Source: CAD feature listing. Evaluate the final solid. Frame: model axes, mm. A direction names the side the tool comes from. Give positions to 0.01 mm unless a question says otherwise; leave off trailing zeros. Write each loop counter-clockwise with the first axis right and the second up, starting at its lowest first coordinate (ties: lowest second). Pieces come first, ordered by that corner, then holes. Notation, with made-up numbers: (54, -37) -> (107, -37) arc R20 ccw to (107, -25) -> close; hole circle Ø3 at (34, 87). An arc over 180 degrees is marked (long way). Answer as a JSON object with one key per item and string values. Group by question number.
Item 1: Section query B-B on x = -9.45. Return the cut outline in (y, z).
Item 2: Ray query, probe 1 along Y at (x, z) = (11.55, -0.75); probe 2 along Y at (x, z) = (0.75, -0.7); probe 3 along Y at (x, z) = (-2.5, 0.6). Return the intervals inside material, ascending. Write a range as from..to.
Item 3: Section query C-C on x = -4.75. Return the cut outline in (y, z), plus the area to 3 significant figures.
Item 4: Access query for faces 1 (the face through (-2, -1, 0)), 2 (the face through (-0.292, 22, -1)), 3 (the face through (-13, 0, -1.2)). Directions: +Z, -Z, +X, -X, +Y, -Y. A direction counts if a zero-diameter tool reaches every point of the face in a straight line with its end or side. Return the directions, or none.
Item 5: Pull-direction query (Y, two-part tool) for faces 4 (the face through (0, 32.8, -1)), 5 (the face through (2, -31.334, -1)), 6 (the face through (10, 27, -2.2)); classes: pulls with the +Y half, pulls with the -Y half, needs draft (parallel to the pull), parting line crosses it, or undercut.
Item 6: First-contact query: pin 1 Ø0.6 at (x, z) = (0.5, -0.5) entering from -Y; pin 2 Ø10 at (x, y) = (1.5, -23) entering from +Z; pin 3 Ø4 at (x, y) = (-2, -22) entering from -Z; pin 4 Ø1.9 at (x, y) = (0.5, 0) entering from +Z. Flat tips, straight axial feed; report the tip coordinate or a pass-through.
from build123d import *

# Parameters (mm, degrees)
SKETCH_2_W          = 29.1
SKETCH_2_H          = 67.8
EXTRUDE_1_DEPTH     = 0.8
SKETCH_3_W          = 29.1
SKETCH_3_H          = 65.6
EXTRUDE_2_DEPTH     = 1.2
SKETCH_4_R          = 1.4
SKETCH_4_W          = 7.042
SKETCH_4_H          = 18.5736
SKETCH_4_W_2        = 4.2
SKETCH_4_H_2        = 8.9
SKETCH_4_W_3        = 8.32
SKETCH_4_H_3        = 15.7
CUT_EXTRUDE_1_DEPTH = 37.944722221
SKETCH_5_R          = 2.1
SKETCH_5_R_2        = 1.1
SKETCH_5_R_3        = 1
EXTRUDE_3_DEPTH     = 1
SKETCH_6_W          = 1
SKETCH_6_H          = 65.6
EXTRUDE_4_DEPTH     = 1
CHAMFER_1_SIZE      = 1
CHAMFER_3_SIZE      = 1
SKETCH_7_W          = 9.042
SKETCH_7_H          = 20.5736
SKETCH_7_W_2        = 6.2
SKETCH_7_H_2        = 10.9
SKETCH_7_W_3        = 10.32
SKETCH_7_H_3        = 17.7
CUT_EXTRUDE_2_DEPTH = 0.8
FILLET_3_R          = 0.8
FILLET_4_R          = 0.8
FILLET_5_R          = 0.8
SKETCH_8_R          = 1.4
CUT_EXTRUDE_3_DEPTH = 37.944722221
CHAMFER_4_SIZE      = 0.6
FILLET_6_R          = 1.6


with BuildPart() as part:
    # Эскиз2 → Бобышка-Вытянуть1 (new body)
    with BuildSketch(Plane.XY):
        Rectangle(SKETCH_2_W, SKETCH_2_H)
    extrude(amount=EXTRUDE_1_DEPTH)

    # Эскиз3 → Бобышка-Вытянуть2 (add)
    with BuildSketch(Plane(origin=(0, 0, 0), x_dir=(-1, 0, 0), z_dir=(0, 0, -1))):
        Rectangle(SKETCH_3_W, SKETCH_3_H)
    extrude(amount=EXTRUDE_2_DEPTH)

    # Эскиз4 → Вырез-Вытянуть1 (cut, through all)
    with BuildSketch(Plane.XY.offset(0.8)):
        with Locations((-9.45, -27.9)):
            Circle(SKETCH_4_R)
        with Locations((11.55, -27.9)):
            Circle(SKETCH_4_R)
        with Locations((11.55, 27.9)):
            Circle(SKETCH_4_R)
        with Locations((-9.45, 27.9)):
            Circle(SKETCH_4_R)
        with Locations((3.229, 22.395)):
            Rectangle(SKETCH_4_W, SKETCH_4_H)
        with Locations((0.55, -0.961534596)):
            Rectangle(SKETCH_4_W_2, SKETCH_4_H_2)
        with Locations((1.86, -23.483733333)):
            Rectangle(SKETCH_4_W_3, SKETCH_4_H_3)
    extrude(amount=-CUT_EXTRUDE_1_DEPTH, mode=Mode.SUBTRACT)

    # Эскиз5 → Бобышка-Вытянуть3 (add)
    # profile 1 of 4: a face of its own
    with BuildSketch(Plane(origin=(0, 0, -1.2), x_dir=(-1, 0, 0), z_dir=(0, 0, -1))):
        with Locations((-11.55, 27.9)):
            Circle(SKETCH_5_R)
        with Locations((-11.55, 27.9)):
            Circle(SKETCH_5_R_2, mode=Mode.SUBTRACT)
    # profile 2 of 4: a face of its own
    with BuildSketch(Plane(origin=(0, 0, -1.2), x_dir=(-1, 0, 0), z_dir=(0, 0, -1))):
        with Locations((-11.55, -27.9)):
            Circle(SKETCH_5_R)
        with Locations((-11.55, -27.9)):
            Circle(SKETCH_5_R_2, mode=Mode.SUBTRACT)
    # profile 3 of 4: a face of its own
    with BuildSketch(Plane(origin=(0, 0, -1.2), x_dir=(-1, 0, 0), z_dir=(0, 0, -1))):
        with Locations((9.45, 27.9)):
            Circle(SKETCH_5_R)
        with Locations((9.45, 27.9)):
            Circle(SKETCH_5_R_3, mode=Mode.SUBTRACT)
    # profile 4 of 4: a face of its own
    with BuildSketch(Plane(origin=(0, 0, -1.2), x_dir=(-1, 0, 0), z_dir=(0, 0, -1))):
        with Locations((9.45, -27.9)):
            Circle(SKETCH_5_R)
        with Locations((9.45, -27.9)):
            Circle(SKETCH_5_R_3, mode=Mode.SUBTRACT)
    extrude(amount=EXTRUDE_3_DEPTH)

    # Эскиз6 → Бобышка-Вытянуть4 (add)
    with BuildSketch(Plane(origin=(0, 0, -1.2), x_dir=(-1, 0, 0), z_dir=(0, 0, -1))):
        with Locations((11.95, 0)):
            Rectangle(SKETCH_6_W, SKETCH_6_H)
    extrude(amount=EXTRUDE_4_DEPTH)

    # Фаска1
    chamfer_1_edges = [part.edges().sort_by_distance(p)[0] for p in [
        (-11.95, -32.8, -2.2),
        (-11.95, 32.8, -2.2),
    ]]
    chamfer(chamfer_1_edges, length=CHAMFER_1_SIZE)

    # Фаска3
    chamfer_3_edges = [part.edges().sort_by_distance(p)[0] for p in [
        (-11.45, -30.670156212, -1.2),
        (-11.45, 30.670156212, -1.2),
        (-11.45, 0, -1.2),
    ]]
    chamfer(chamfer_3_edges, length=CHAMFER_3_SIZE - 0.0001)  # a hair under: the kernel refuses the full size

    # Эскиз7 → Вырез-Вытянуть2 (cut)
    with BuildSketch(Plane.XY.offset(0.8)):
        with Locations((3.229, 22.395)):
            Rectangle(SKETCH_7_W, SKETCH_7_H)
        with Locations((0.55, -0.961534596)):
            Rectangle(SKETCH_7_W_2, SKETCH_7_H_2)
        with Locations((1.86, -23.483733333)):
            Rectangle(SKETCH_7_W_3, SKETCH_7_H_3)
    extrude(amount=-CUT_EXTRUDE_2_DEPTH, mode=Mode.SUBTRACT)

    # Скругление3
    fillet_3_edges = [part.edges().sort_by_distance(p)[0] for p in [
        (3.229, 12.1082, 0.8),
        (7.75, 22.395, 0.8),
        (3.229, 32.6818, 0.8),
        (-1.292, 22.395, 0.8),
    ]]
    fillet(fillet_3_edges, radius=FILLET_3_R - 0.0001)  # a hair under: the kernel refuses the full size

    # Скругление4
    fillet_4_edges = [part.edges().sort_by_distance(p)[0] for p in [
        (0.55, -6.411534596, 0.8),
        (-2.55, -0.961534596, 0.8),
        (0.55, 4.488465404, 0.8),
        (3.65, -0.961534596, 0.8),
    ]]
    fillet(fillet_4_edges, radius=FILLET_4_R - 0.0001)  # a hair under: the kernel refuses the full size

    # Скругление5
    fillet_5_edges = [part.edges().sort_by_distance(p)[0] for p in [
        (1.86, -32.333733333, 0.8),
        (-3.3, -23.483733333, 0.8),
        (1.86, -14.633733333, 0.8),
        (7.02, -23.483733333, 0.8),
    ]]
    fillet(fillet_5_edges, radius=FILLET_5_R - 0.0001)  # a hair under: the kernel refuses the full size

    # Эскиз8 → Вырез-Вытянуть3 (cut, through all)
    with BuildSketch(Plane.XY.offset(-1.2)):
        with Locations((11.55, 27.9)):
            Circle(SKETCH_8_R)
        with Locations((-9.45, -27.9)):
            Circle(SKETCH_8_R)
        with Locations((11.55, -27.9)):
            Circle(SKETCH_8_R)
        with Locations((-9.45, 27.9)):
            Circle(SKETCH_8_R)
    extrude(amount=-CUT_EXTRUDE_3_DEPTH, mode=Mode.SUBTRACT)

    # Фаска4
    chamfer_4_edges = [part.edges().sort_by_distance(p)[0] for p in [
        (10.15, -27.9, 0.8),
        (10.15, 27.9, 0.8),
        (-10.85, 27.9, 0.8),
        (-10.85, -27.9, 0.8),
    ]]
    chamfer(chamfer_4_edges, length=CHAMFER_4_SIZE)

    # Скругление6
    fillet_6_edges = [part.edges().sort_by_distance(p)[0] for p in [
        (-14.55, 0, 0.8),
    ]]
    fillet(fillet_6_edges, radius=FILLET_6_R)


solid = part.part
Worked answers:
{
 "1": {"outline": "(-33.9, 0) -> (-32.8, 0) -> (-32.8, -1.2) -> (-30, -1.2) -> (-30, -2.2) -> (-29.3, -2.2) -> (-29.3, 0.2) -> (-29.9, 0.8) -> (-33.9, 0.8) -> close; (-26.5, -2.2) -> (-25.8, -2.2) -> (-25.8, -1.2) -> (25.8, -1.2) -> (25.8, -2.2) -> (26.5, -2.2) -> (26.5, 0.2) -> (25.9, 0.8) -> (-25.9, 0.8) -> (-26.5, 0.2) -> close; (29.3, -2.2) -> (30, -2.2) -> (30, -1.2) -> (32.8, -1.2) -> (32.8, 0) -> (33.9, 0) -> (33.9, 0.8) -> (29.9, 0.8) -> (29.3, 0.2) -> close"},
 "2": {"probe 1": "-32.8..-29.3, -26.5..26.5, 29.3..32.8", "probe 2": "-32.8..-31.33, -15.63..-5.41, 3.49..13.11, 31.68..32.8", "probe 3": "-33.9..-32.6, -14.36..-6.68, 4.76..33.9"},
 "3": {"outline": "(-33.9, 0) -> (-32.8, 0) -> (-32.8, -1.2) -> (32.8, -1.2) -> (32.8, 0) -> (33.9, 0) -> (33.9, 0.8) -> (-33.9, 0.8) -> close", "area": "133 mm^2"},
 "4": {"face 1": "+Z", "face 2": "+Z, -Z", "face 3": "-Z, -X, +Y, -Y"},
 "5": {"face 4": "pulls with the +Y half", "face 5": "undercut", "face 6": "needs draft"},
 "6": {"pin 1": "y = -32.8", "pin 2": "z = 0.53", "pin 3": "z = -1.2", "pin 4": "through"}
}
